Geometry: see drawing. Coordinates: mm, zero at the bounding-box minimum. A direction names the side the tool comes from. Give positions to 0.01 mm unless a question says otherwise; leave off trailing zeros. Write each loop counter-clockwise with the first axis right and the second up, starting at its lowest first coordinate (ties: lowest second). Pieces come first, ordered by that corner, then holes. Notation, with made-up numbers: (24, 53.5) -> (35, 53.5) arc R12 cw to (35, 67.5) -> close; hole circle Ø9 at (78.25, -26). An arc over 180 degrees is marked (long way). Use one line per item in the form item = value. Start each with the question number.
(1) Cut plane C-C, the plane x = 124. Output: boundary loops of the cut face in (y, z).
(2) Cut plane B-B, the plane y = 9.25. Output: boundary loops of the cut face in (x, z).
(3) Material intervals for line 1 along X through (y, z) = (4.75, 4); line 2 along X through (y, z) = (2.25, 3); line 3 along Y through (x, z) = (53.5, 6), sorted ascending. Write a range as from..to.
(4) Set-up query: the marked faces 4 and 5. Return all of +Z, -Z, +X, -X, +Y, -Y with unobstructed straight access to the full face (end or side cutting, diameter ignored); none if empty.
(5) Cut plane A-A, the plane z = 6. Output: boundary loops of the cut face in (x, y).
(6) Cut plane D-D, the plane y = 18.25. Output: boundary loops of the cut face in (x, z).
(7) Draft query along X for the marked faces 1, 2 and 3. Return one class per face: pulls with the +X half, pulls with the -X half, needs draft (parallel to the pull), parting line crosses it, or undercut.
(8) First-contact query: P1, Ø3, axis at x = 102, y = 18.5, coming from the -Z side; P2, Ø5, axis at x = 38.5, y = 16.5, coming from the +Z side; P3, Ø3, axis at x = 31.5, y = 23, coming from the +Z side. Flat tips, straight axial feed; report the tip coordinate or a pass-through.
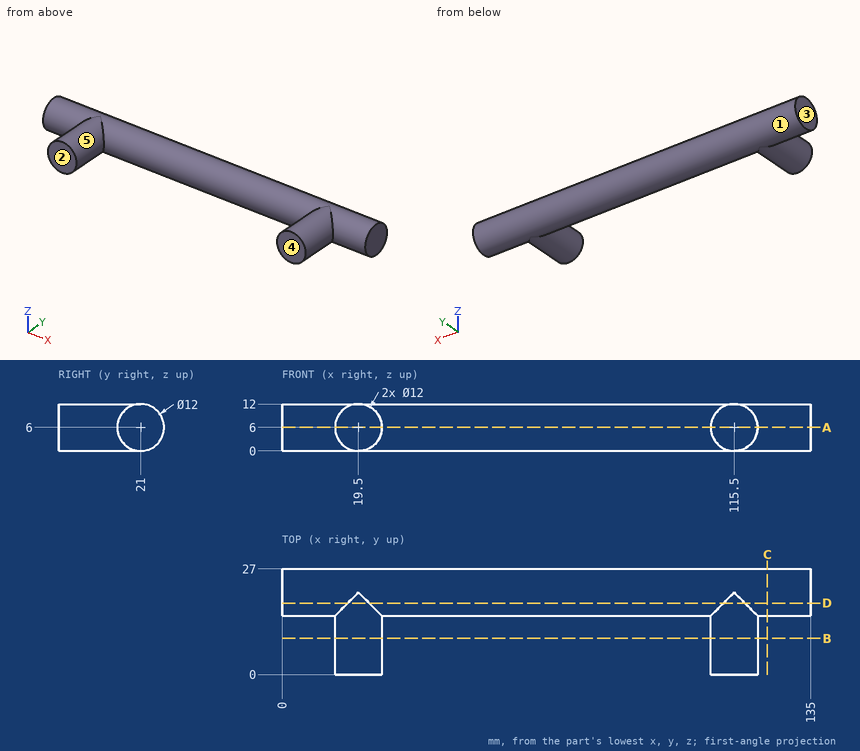
Geometry says:
q1.outline = circle Ø12 at (21, 6)
q2.outline = circle Ø12 at (19.5, 6); circle Ø12 at (115.5, 6)
q3.line_1 = 13.84..25.16, 109.84..121.16
q3.line_2 = 14.3..24.7, 110.3..120.7
q3.line_3 = 15..27
q4.face_4 = +Z, -Z, +X, -X, -Y
q4.face_5 = -Y
q5.outline = (0, 15) -> (13.5, 15) -> (13.5, 0) -> (25.5, 0) -> (25.5, 15) -> (109.5, 15) -> (109.5, 0) -> (121.5, 0) -> (121.5, 15) -> (135, 15) -> (135, 27) -> (0, 27) -> close
q6.outline = (0, 0.67) -> (16.75, 0.67) arc R6 ccw to (22.25, 0.67) -> (112.75, 0.67) arc R6 ccw to (118.25, 0.67) -> (135, 0.67) -> (135, 11.33) -> (118.25, 11.33) arc R6 ccw to (112.75, 11.33) -> (22.25, 11.33) arc R6 ccw to (16.75, 11.33) -> (0, 11.33) -> close
q7.face_1 = undercut
q7.face_2 = needs draft
q7.face_3 = pulls with the -X half
q8.P1 = 0.08
q8.P2 = 11.66
q8.P3 = 11.98
